```python
from build123d import *

# Parameters (mm, degrees)
SKETCH1_R                = 10.25
BOSS_EXTRUDE1_DEPTH      = 7
SKETCH2_R                = 3.75
CUT_EXTRUDE1_DEPTH       = 2
BOSS_EXTRUDE3_START      = -7
BOSS_EXTRUDE3_DEPTH      = 7
SKETCH11_R               = 2.25
CUT_EXTRUDE3_DEPTH       = 30
CUT_EXTRUDE4_DEPTH       = 3
SKETCH15_R               = 10.25
BOSS_EXTRUDE4_DEPTH      = 65
BOSS_EXTRUDE5_DEPTH      = 58
CUT_EXTRUDE5_DEPTH       = 44
CUT_EXTRUDE5_DEPTH_BACK  = 34
BOSS_EXTRUDE6_DEPTH      = 15
BOSS_EXTRUDE6_DEPTH_BACK = 20
SKETCH20_R               = 10.25
SKETCH21_R               = 3.75
CUT_EXTRUDE6_DEPTH       = 92


with BuildPart() as part:
    # Sketch1 → Boss-Extrude1 (new body)
    with BuildSketch(Plane.XY):
        Circle(SKETCH1_R)
    extrude(amount=BOSS_EXTRUDE1_DEPTH)

    # Sketch2 → Cut-Extrude1 (cut)
    with BuildSketch(Plane(origin=(0, 0, 0), x_dir=(-1, 0, 0), z_dir=(0, 0, -1))):
        with Locations((0.204827132, 0.201115052)):
            Circle(SKETCH2_R)
    cut_extrude1 = extrude(amount=-CUT_EXTRUDE1_DEPTH, mode=Mode.SUBTRACT)

    # Sketch4 → Boss-Extrude3 (add)
    with BuildSketch(Plane.XY.offset(7).offset(BOSS_EXTRUDE3_START)):
        with BuildLine():
            add(Edge.make_bspline(
                [(-46.64048221, 0), (-34.962013149, 28.10744238), (-2.004119339, 10.052164228)],
                knots=[0, 0, 0, 1, 1, 1], degree=2))
            Line((-46.64048221, 0), (-37.28232369, -4.481971191))
            add(Edge.make_bspline(
                [(-10.196546661, 1.045435881), (-26.46828973, 10.703347347), (-37.28232369, -4.481971191)],
                knots=[0, 0, 0, 1, 1, 1], degree=2))
            ThreePointArc((-10.196546661, 1.045435881), (-7.58250299, 6.896966609), (-2.004119339, 10.052164228))
        make_face()
    boss_extrude3 = extrude(amount=BOSS_EXTRUDE3_DEPTH)

    # Sketch11 → Cut-Extrude3 (cut)
    with BuildSketch(Plane(origin=(-8.702296632, -18.170012234, 0), x_dir=(0, 0, 1), z_dir=(-0.4319519366403788, -0.9018966262452843, 0))):
        with Locations(Location((3.5, 35.498805819, 0), (0, 0, 270))):
            Circle(SKETCH11_R)
    cut_extrude3 = extrude(amount=-CUT_EXTRUDE3_DEPTH, mode=Mode.SUBTRACT)

    # Sketch13 → Cut-Extrude4 (cut)
    with BuildSketch(Plane(origin=(0, 0, 0), x_dir=(-1, 0, 0), z_dir=(0, 0, -1))):
        Polygon((34.379239122, 13.872575937), (31.676706965, 12.578232477), (34.770203183, 6.119148571), (37.47273534, 7.41349203), align=None)
    cut_extrude4 = extrude(amount=-CUT_EXTRUDE4_DEPTH, mode=Mode.SUBTRACT)

    # Sketch15 → Boss-Extrude4 (add)
    with BuildSketch(Plane.XY.offset(7)):
        with Locations(Location((0, 0, 0), (0, 0, 174.146009255))):
            Circle(SKETCH15_R)
    extrude(amount=BOSS_EXTRUDE4_DEPTH)

    # Mirror1: Cut-Extrude1, Boss-Extrude3, Cut-Extrude3, Cut-Extrude4 across plane
    add(cut_extrude1.mirror(Plane.XY.offset(36)), mode=Mode.SUBTRACT)
    add(boss_extrude3.mirror(Plane.XY.offset(36)))
    add(cut_extrude3.mirror(Plane.XY.offset(36)), mode=Mode.SUBTRACT)
    add(cut_extrude4.mirror(Plane.XY.offset(36)), mode=Mode.SUBTRACT)

    # Sketch18 → Boss-Extrude5 (add)
    with BuildSketch(Plane.XY.offset(7)):
        with BuildLine():
            Line((-46.64048221, 0), (-37.28232368, -4.481971176))
            add(Edge.make_bspline(
                [(-37.28232368, -4.481971176), (-26.468289723, 10.703347342), (-10.196546661, 1.045435881)],
                knots=[0, 0, 0, 1, 1, 1], degree=2))
            ThreePointArc((-10.196546661, 1.045435881), (-7.58250299, 6.896966609), (-2.004119339, 10.052164228))
            add(Edge.make_bspline(
                [(-2.004119339, 10.052164228), (-34.962013149, 28.10744238), (-46.64048221, 0)],
                knots=[0, 0, 0, 1, 1, 1], degree=2))
        make_face()
    extrude(amount=BOSS_EXTRUDE5_DEPTH)

    # Sketch19 → Cut-Extrude5 (cut, two sides: drawn at the far end of the back side and taken through both)
    with BuildSketch(Plane(origin=(0, 0, 0), x_dir=(1, 0, 0), z_dir=(0, 1, 0)).offset(-CUT_EXTRUDE5_DEPTH_BACK)):
        with BuildLine():
            Line((-56.84662667, -7), (-30.196546661, -7))
            ThreePointArc((-30.196546661, -7), (-16.054411038, -12.857864376), (-10.196546661, -27))
            Line((-10.196546661, -27), (-10.25, -45))
            ThreePointArc((-10.25, -45), (-16.107864376, -59.142135624), (-30.25, -65))
            Line((-30.25, -65), (-56.84662667, -65))
            Line((-56.84662667, -65), (-56.84662667, -7))
        make_face()
    extrude(amount=CUT_EXTRUDE5_DEPTH + CUT_EXTRUDE5_DEPTH_BACK, mode=Mode.SUBTRACT)

    # Sketch20 → Boss-Extrude6 (add, two sides: drawn at the far end of the back side and taken through both)
    with BuildSketch(Plane.XY.offset(36).offset(-BOSS_EXTRUDE6_DEPTH_BACK)):
        Circle(SKETCH20_R)
    extrude(amount=BOSS_EXTRUDE6_DEPTH + BOSS_EXTRUDE6_DEPTH_BACK)

    # Sketch21 → Cut-Extrude6 (cut)
    with BuildSketch(Plane.XY.offset(70)):
        with Locations(Location((-0.204827132, 0.201115052, 0), (0, 0, 180))):
            Circle(SKETCH21_R)
    extrude(amount=-CUT_EXTRUDE6_DEPTH, mode=Mode.SUBTRACT)


solid = part.part
```
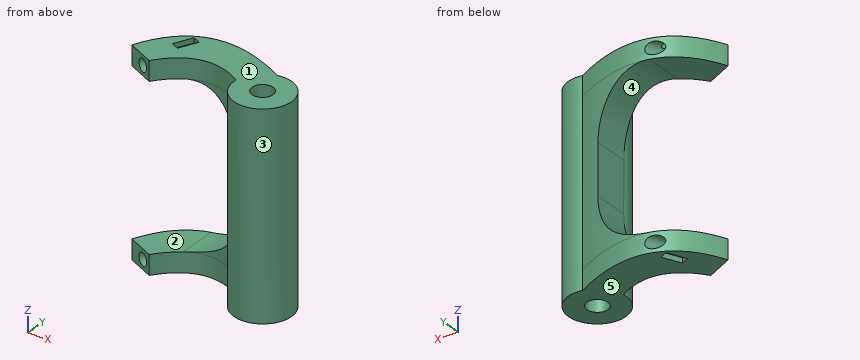
Design review of the part built by this model. Coordinates are the model's own, in mm. Face numbers are marked on the shaded views. A direction names the side the tool comes from. Give positions to 0.01 mm unless a question says otherwise; leave off trailing zeros. Write each loop counter-clockwise with the first axis right and the second up, starting at its lowest first coordinate (ties: lowest second). Pieces come first, ordered by that corner, then holes.
(1) Tool access review of the marked faces 1 and 2: name each direction out of +Z, -Z, +X, -X, +Y, -Y from which nothing blocks a thin tool from reaching the whole face with its end or side.
Checked values:
face 1: +Z, +X, -X, +Y, -Y
face 2: -X, +Y, -Y
(2) Mouldability with a two-part tool opening along Z and no side actions: class the marked faces 3, 4 and 5 as +Z half, -Z half, draft (parallel to the pull), parting line (faces both ways), or undercut.
Checked values:
face 3: draft
face 4: undercut
face 5: -Z half
(3) Wall thickness on line 1 along X through (y, z) = (-0.5, 6); line 2 along Z through (x, y) = (-43, 3.5); line 3 along X through (y, z) = (0, 61.5): over which ranges is each line inside the solid? List them lowest first.
Checked values:
line 1: x = -45.6 to -33.93, -10.24 to -3.89, 3.48 to 10.24
line 2: z = 0 to 7, 65 to 72
line 3: x = -10.25 to -3.95, 3.54 to 10.25
(4) Add section A-A (x = 0). Give the boundary of the cut face in (y, z), and give its area (3 significant figures).
Checked values:
outline: (-10.25, 0) - (-3.54, 0) - (-3.54, 72) - (-10.25, 72) - close; (3.95, 0) - (10.25, 0) - (10.25, 72) - (3.95, 72) - close
area: 937 mm2
(5) Clearance check with flat-ended pins moving along their axes: pin 1 Ø4 at (x, z) = (-2, 36) entering from +Y; pin 2 Ø8 at (y, z) = (-4.5, 39) entering from -X; pin 3 Ø1.5 at (x, z) = (2, 41) entering from +Y. State where each tip first meets the part, or that it passes through.
Checked values:
pin 1: stops at y = 11.11
pin 2: stops at x = -10.24
pin 3: stops at y = 10.17
